Read the model definition and answer for the solid it produces. Units are mm, in the model's axes. A direction names the side the tool comes from. Round coordinates to 2 decimals unless told otherwise and drop trailing zeros. Order: outer loops, then holes, each group sorted by start corner. A loop starts at its lowest first (then second) coordinate and runs counter-clockwise, first axis right, second up. Notation, with made-up numbers: M 15.25,57.25 L 25.25,57.25 A4 cw 25.25,64.25 Z; hole C 73.5,4 d9. An arc over 180 degrees is marked long. Answer as CSV lines item,"result".
Autodesk Inventor part; units mm, degrees
ref_plane "YZ Plane" through (0, 0, 0) normal (1, 0, 0) x (0, 1, 0)
ref_plane "XZ Plane" through (0, 0, 0) normal (0, 1, 0) x (-1, 0, 0)
ref_plane "XY Plane" through (0, 0, 0) normal (0, 0, 1) x (1, 0, 0)
sketch "Sketch1" plane through (0, 0, 0) normal (0, 0, 1) x (1, 0, 0)
  line L0 (-65.675, -42.2) -> (65.675, -42.2)
  line L1 (65.675, -42.2) -> (65.675, 42.2)
  line L2 (65.675, 42.2) -> (-65.675, 42.2)
  line L3 (-65.675, 42.2) -> (-65.675, -42.2)
  line L4 (-65.675, -42.2) -> (65.675, 42.2) construction
  line L5 (65.675, -42.2) -> (-65.675, 42.2) construction
  point P0 (0, 0)
  dimension "d0" = 131.35
  dimension "d1" = 84.4
extrude "Extrusion1" add sketch "Sketch1" along normal blind 32.7
sketch "Sketch2" plane through (0, 0, 32.7) normal (0, 0, 1) x (1, 0, 0)
  line L0 (65.675, 42.2) -> (-65.675, 42.2)
  line L1 (-65.675, -42.2) -> (65.675, -42.2)
  line L2 (-30.675, 42.2) -> (35.675, 42.2)
  line L3 (35.675, 42.2) -> (35.675, 22.2)
  line L4 (35.675, 22.2) -> (-30.675, 22.2)
  line L5 (-30.675, 22.2) -> (-30.675, 42.2)
  line L6 (-30.675, -42.2) -> (35.675, -42.2)
  line L7 (35.675, -42.2) -> (35.675, -22.2)
  line L8 (35.675, -22.2) -> (-30.675, -22.2)
  line L9 (-30.675, -22.2) -> (-30.675, -42.2)
  line L10 (65.675, -42.2) -> (65.675, 42.2)
  line L11 (-65.675, 42.2) -> (-65.675, -42.2)
  line L12 (65.675, 42.2) -> (55.675, 42.2)
  line L13 (55.675, 42.2) -> (55.675, -42.2)
  line L14 (55.675, -42.2) -> (65.675, -42.2)
  line L15 (65.675, -42.2) -> (65.675, 42.2)
  line L16 (-65.675, 42.2) -> (-55.675, 42.2)
  line L17 (-55.675, 42.2) -> (-55.675, -42.2)
  line L18 (-55.675, -42.2) -> (-65.675, -42.2)
  line L19 (-65.675, -42.2) -> (-65.675, 42.2)
  point P0 (0, 0)
  dimension "d5" = 20
  dimension "d6" = 20
  dimension "d7" = 30
  dimension "d8" = 35
  dimension "d9" = 35
  dimension "d10" = 10
  dimension "d11" = 10
extrude "Extrusion2" cut sketch "Sketch2" against normal blind 28 contours L10 L1 L13 L0 | L3 L4 L5 L0 | L1 L9 L8 L7 | L17 L1 L11 L0
chamfer "Chamfer1" distance 18.75 angle 45 4 edges at (-43.175, -42.2, 32.7) (45.675, -42.2, 32.7) (45.675, 42.2, 32.7) (-43.175, 42.2, 32.7)
sketch "Sketch3" plane through (0, 0, 4.7) normal (0, 0, 1) x (1, 0, 0)
  circle A0 centre (-6.675, 35.2) radius 3
  circle A1 centre (-10.675, -35.2) radius 3
  circle A2 centre (13.325, -35.2) radius 3
  line L0 (-30.675, 42.2) -> (35.675, 42.2)
  line L1 (35.675, -42.2) -> (55.675, -42.2)
  line L2 (-65.675, -42.2) -> (-65.675, 42.2)
  point P0 (0, 0)
  dimension "d17" = 24
  dimension "d18" = 20
  dimension "d19" = 70.4
  dimension "d20" = 7
  dimension "d21" = 84.4
  dimension "d22" = 6
  dimension "d23" = 6
  dimension "d24" = 6
  dimension "d25" = 55
  dimension "d26" = 0
extrude "Extrusion3" cut sketch "Sketch3" against normal blind 28
equation "\"d6\" = d5"
equation "\"d9\" = d8"
equation "\"d20\" = -0.5 * d19 + 0.5 * d21"
equation "\"d23\" = d22"
equation "\"d24\" = d22"
properties part number "FuseBox_04980933.X"
Item 1: A cutting plane is placed at B-B, the plane y = -35.2. Determine the outline of the cut face in (x, z) (3 decimals).
Ans:
outline,"M -65.675,0 L -13.675,0 L -13.675,4.7 L -30.675,4.7 L -30.675,20.95 L -55.675,20.95 L -55.675,4.7 L -65.675,4.7 Z; M -7.675,0 L 10.325,0 L 10.325,4.7 L -7.675,4.7 Z; M 16.325,0 L 65.675,0 L 65.675,4.7 L 55.675,4.7 L 55.675,20.95 L 35.675,20.95 L 35.675,4.7 L 16.325,4.7 Z"
Item 2: A tool of negligible diameter and unlimited length cuts with its end or side. For faces 4 (the face through (3, 22.2, 19)), 5 (the face through (35.675, -30, 16)), 6 (the face through (-43.35, 32.69, 23.46)), 7 (the face through (55.675, 1, 19)), 8 (the face through (-61, 1, 4.7)), from which of +Z, -Z, +X, -X, +Y, -Y can it reach the whole face along a straight path? Write none if from no direction.
Ans:
face 4,"+Z, +Y"
face 5,"+Z, -Y"
face 6,"+Z, +X, -X, +Y"
face 7,"+Z, +X, +Y, -Y"
face 8,"+Z, -X, +Y, -Y"
Item 3: A cutting plane is placed at A-A, the plane y = 35.2. Determine the outline of the cut face in (x, z) (3 decimals), and give its area (3 significant figures).
Ans:
outline,"M -65.675,0 L -9.675,0 L -9.675,4.7 L -30.675,4.7 L -30.675,20.95 L -55.675,20.95 L -55.675,4.7 L -65.675,4.7 Z; M -3.675,0 L 65.675,0 L 65.675,4.7 L 55.675,4.7 L 55.675,20.95 L 35.675,20.95 L 35.675,4.7 L -3.675,4.7 Z"
area,"1,320 mm2"
Item 4: A cutting plane is placed at D-D, the plane x = 2.5. Determine the outline of the cut face in (y, z), and give its area (3 significant figures).
Ans:
outline,"M -42.2,0 L 42.2,0 L 42.2,4.7 L 22.2,4.7 L 22.2,32.7 L -22.2,32.7 L -22.2,4.7 L -42.2,4.7 Z"
area,"1,640 mm2"
Item 5: A cutting plane is placed at C-C, the plane z = 19. Determine the outline of the cut face in (x, y) (3 decimals).
Ans:
outline,"M -55.675,-37.15 L -30.675,-37.15 L -30.675,-22.2 L 35.675,-22.2 L 35.675,-37.15 L 55.675,-37.15 L 55.675,37.15 L 35.675,37.15 L 35.675,22.2 L -30.675,22.2 L -30.675,37.15 L -55.675,37.15 Z"
Item 6: Determine the mould class of faces 1 (the face through (2, -32, 4.7)), 2 (the face through (-11.066, -32.226, 2.383)), 3 (the face through (-1, -42.2, 4)) for opening direction Y: +Y half, -Y half, draft (parallel to the pull), parting line (faces both ways), or undercut.
Ans:
face 1,"draft"
face 2,"undercut"
face 3,"-Y half"
Item 7: Find the intervals of material crossed by probe 1 along X at (y, z) = (26, 20) (3 decimals); probe 2 along Y at (x, z) = (-0.5, 5.5); probe 3 along Z at (x, y) = (-3, 23), in increasing order. Write a range as [from, to].
Ans:
probe 1,"[-55.675, -30.675], [35.675, 55.675]"
probe 2,"[-22.2, 22.2]"
probe 3,"[0, 4.7]"
Item 8: Flat-ended cylindrical pins translate along their axes: pin 1 (8.5 mm diameter, centred on x = -7, z = 20, fed in from -Y); pin 2 (6 mm diameter, centred on x = -9.5, y = -27.5, fed in from +Z); pin 3 (12 mm diameter, centred on y = -28, z = 16, fed in from -X) (3 decimals); pin 4 (1.5 mm diameter, centred on x = -38.5, y = -30, fed in from -Z). Find the tip coordinate at first contact, or state that the pin passes through.
Ans:
pin 1,"y = -22.2"
pin 2,"z = 4.7"
pin 3,"x = -55.675"
pin 4,"z = 0"
